```python
from build123d import *

# Parameters (mm, degrees)
SKETCH1_R           = 11
SKETCH1_R_2         = 2.1
BOSS_EXTRUDE1_DEPTH = 8
SKETCH2_R           = 8
SKETCH2_R_2         = 2.1
BOSS_EXTRUDE2_DEPTH = 4


with BuildPart() as part:
    # Sketch1 → Boss-Extrude1 (new body)
    with BuildSketch(Plane.XY):
        Polygon((-20, 20), (20, 20), (20, -21), (6.5, -41), (-6.5, -41), (-20, -21), align=None)
        Circle(SKETCH1_R, mode=Mode.SUBTRACT)
        with Locations((0, -35)):
            Circle(SKETCH1_R_2, mode=Mode.SUBTRACT)
        with Locations((0, -25)):
            Circle(SKETCH1_R_2, mode=Mode.SUBTRACT)
    extrude(amount=BOSS_EXTRUDE1_DEPTH)

    # Sketch2 → Boss-Extrude2 (add)
    with BuildSketch(Plane.XY.offset(8)):
        Polygon((20, -21), (20, 20), (-20, 20), (-20, -21), (-6.5, -41), (6.5, -41), align=None)
        Circle(SKETCH2_R, mode=Mode.SUBTRACT)
        with Locations((0, -35)):
            Circle(SKETCH2_R_2, mode=Mode.SUBTRACT)
        with Locations((0, -25)):
            Circle(SKETCH2_R_2, mode=Mode.SUBTRACT)
    extrude(amount=BOSS_EXTRUDE2_DEPTH)


solid = part.part
```
Verification items for the finished model (mm, model axes). A direction names the side the tool comes from. Round coordinates to 2 decimals unless told otherwise and drop trailing zeros. Order: outer loops, then holes, each group sorted by start corner. A loop starts at its lowest first (then second) coordinate and runs counter-clockwise, first axis right, second up.
1) Tool access check on faces 1 (the cylindrical face through (-2.38, -10.74, 3.94)), 2 (the flat face through (-20, 0, 6)). Record the directions out of +Z, -Z, +X, -X, +Y, -Y that give a thin tool (end or side, any length) a straight path to the whole face; none if there is none.
Geometry says:
face 1: -Z
face 2: +Z, -Z, -X, +Y, -Y
2) Depth check by flat-ended pin: pin 1 (2 mm diameter, centred on x = -15, y = -33, fed in from -Z); pin 2 (21 mm diameter, centred on x = 0, y = 0, fed in from +Z); pin 3 (4 mm diameter, centred on y = -26, z = 3.5, fed in from +X) (3 decimals); pin 4 (4 mm diameter, centred on x = -15.5, z = 8, fed in from -Y). Enter the tip coordinate at first touch or a pass-through.
Geometry says:
pin 1: passes through
pin 2: stops at z = 12
pin 3: stops at x = 17.975
pin 4: stops at y = -30.63
3) Draft check along Y on faces 3 (the flat face through (20, -1, 6)), 4 (the flat face through (0, -41, 6)), 5 (the cylindrical face through (1.13, -23.23, 5.92)). Enter one of: +Y half, -Y half, draft (parallel to the pull), parting line (faces both ways), or undercut.
Geometry says:
face 3: draft
face 4: -Y half
face 5: undercut
4) Cross-section at C-C, the plane z = 9.75. Record the cut outline in (x, y).
Geometry says:
outline: (-20, -21) - (-6.5, -41) - (6.5, -41) - (20, -21) - (20, 20) - (-20, 20) - close; hole circle Ø16 at (0, 0); hole circle Ø4.2 at (0, -35); hole circle Ø4.2 at (0, -25)
5) Cross-section at A-A, the plane x = 0. Record the cut outline in (y, z).
Geometry says:
outline: (-41, 0) - (-37.1, 0) - (-37.1, 12) - (-41, 12) - close; (-32.9, 0) - (-27.1, 0) - (-27.1, 12) - (-32.9, 12) - close; (-22.9, 0) - (-11, 0) - (-11, 8) - (-8, 8) - (-8, 12) - (-22.9, 12) - close; (8, 8) - (11, 8) - (11, 0) - (20, 0) - (20, 12) - (8, 12) - close
6) Cross-section at B-B, the plane y = 0. Record the cut outline in (x, z).
Geometry says:
outline: (-20, 0) - (-11, 0) - (-11, 8) - (-8, 8) - (-8, 12) - (-20, 12) - close; (8, 8) - (11, 8) - (11, 0) - (20, 0) - (20, 12) - (8, 12) - close
7) Material ranges on line 1 (Y direction, x = 0, z = 6); line 2 (Y direction, x = 0, z = 9.2); line 3 (Y direction, x = 9.5, z = 2.5), recorded low to high.
Geometry says:
line 1: y = -41 to -37.1, -32.9 to -27.1, -22.9 to -11, 11 to 20
line 2: y = -41 to -37.1, -32.9 to -27.1, -22.9 to -8, 8 to 20
line 3: y = -36.56 to -5.55, 5.55 to 20
8) Cross-section at D-D, the plane y = -25. Record the cut outline in (x, z), plus the area to 3 significant figures.
Geometry says:
outline: (-17.3, 0) - (-2.1, 0) - (-2.1, 12) - (-17.3, 12) - close; (2.1, 0) - (17.3, 0) - (17.3, 12) - (2.1, 12) - close
area: 365 mm2
